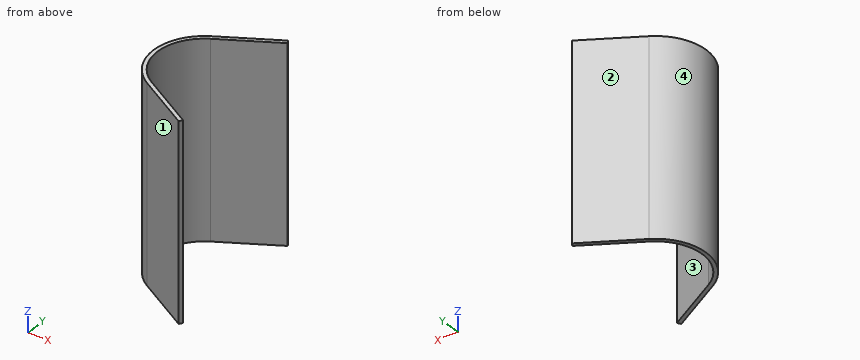
Autodesk Inventor part; units mm, degrees
ref_plane "YZ Plane" through (0, 0, 0) normal (1, 0, 0) x (0, 1, 0)
ref_plane "XZ Plane" through (0, 0, 0) normal (0, 1, 0) x (-1, 0, 0)
ref_plane "XY Plane" through (0, 0, 0) normal (0, 0, 1) x (1, 0, 0)
sketch "Sketch1" plane through (0, 0, 0) normal (0, 0, 1) x (1, 0, 0)
  arc A0 (-3, 5.1962) -> (-3, -5.1962) centre (0, 0) ccw
  line L0 (-3, 5.1962) -> (4, 9.2376)
  line L1 (-3, -5.1962) -> (4, -9.2376)
  line L2 (0, 0) -> (4, 0)
  line L3 (3.75, 9.6706) -> (-3.25, 5.6292)
  arc A1 (-3.25, 5.6292) -> (-3.25, -5.6292) centre (0, 0) ccw
  line L4 (-3.25, -5.6292) -> (3.75, -9.6706)
  line L5 (3.75, 9.6706) -> (4, 9.2376)
  line L6 (4, -9.2376) -> (3.75, -9.6706)
  dimension "d0" = 12
  dimension "d1" = 4
  dimension "d2" = 60
  dimension "d3" = 0.5
extrude "Extrusion1" add sketch "Sketch1" along normal blind 25
properties part number "preanode-screen" material "Stainless Steel"
Can you work these out from the model? Positions are in its coordinate system, mm. Face numbers are marked on the shaded views. Give positions to 0.01 mm unless a question says otherwise; leave off trailing zeros. Order: outer loops, then holes, each group sorted by start corner. A loop starts at its lowest first (then second) coordinate and runs counter-clockwise, first axis right, second up. Notation, with made-up numbers: (42, 7.25) - (79, 7.25) arc R33 cw to (79, 39.25) - close; hole circle Ø4 at (-28.5, 50.25). An arc over 180 degrees is marked (long way). Use a Markdown table: item, result. Add a question column.
Q1. I'm going to push flat-ended pins straight in: pin 1 (1.5 mm diameter, centred on x = 0.5, z = 7, fed in from -Y); pin 2 (5 mm diameter, centred on x = -2, z = 17.5, fed in from +Y); pin 3 (1 mm diameter, centred on x = 1, z = 12, fed in from +Y); pin 4 (1 mm diameter, centred on x = -5, y = -0.5, fed in from +Z). Where does each tip first touch, or does it pass through?
Q2. If we section it at C-C on x = -5: Write out the boundary of the cut face in (y, z).
Q3. If we section it at A-A on z = 18.5: Write out the boundary of the cut face in (x, y), plus the area to 3 significant figures.
Q4. If we section it at B-B on x = 1.5: Write out the boundary of the cut face in (y, z).
Q5. If we section it at D-D on y = 0: Write out the boundary of the cut face in (x, z), plus the area to 3 significant figures.
Q6. If we mould it in two halves opening along Y, with no side actions, what happens to the marked faces 1, 2, 3 and 4? For each: released by +Y, released by -Y, zero draft, split by the parting line, or undercut.
Q7. Please list where these lines run through material, in increasing order: line 1 along Y through (x, z) = (2, 3); line 2 along Y through (x, z) = (0, 12.25); line 3 along X through (y, z) = (7.75, 10.75).
Answers follow:
| question | item | result |
|---|---|---|
| 1 | pin 1 | stops at y = -8.23 |
| 1 | pin 2 | stops at y = 7.79 |
| 1 | pin 3 | stops at y = 8.37 |
| 1 | pin 4 | passes through |
| 2 | outline | (-4.15, 0) - (-3.32, 0) - (-3.32, 25) - (-4.15, 25) - close; (3.32, 0) - (4.15, 0) - (4.15, 25) - (3.32, 25) - close |
| 3 | outline | (-3.25, -5.63) - (3.75, -9.67) - (4, -9.24) - (-3, -5.2) arc R6 cw to (-3, 5.2) - (4, 9.24) - (3.75, 9.67) - (-3.25, 5.63) arc R6.5 ccw to start |
| 3 | area | 14.6 mm^2 |
| 4 | outline | (-8.37, 0) - (-7.79, 0) - (-7.79, 25) - (-8.37, 25) - close; (7.79, 0) - (8.37, 0) - (8.37, 25) - (7.79, 25) - close |
| 5 | outline | (-6.5, 0) - (-6, 0) - (-6, 25) - (-6.5, 25) - close |
| 5 | area | 12.5 mm^2 |
| 6 | face 1 | released by -Y |
| 6 | face 2 | released by +Y |
| 6 | face 3 | undercut |
| 6 | face 4 | split by the parting line |
| 7 | line 1 | y = -8.66 to -8.08, 8.08 to 8.66 |
| 7 | line 2 | y = -7.51 to -6.93, 6.93 to 7.51 |
| 7 | line 3 | x = 0.42 to 1.42 |
